Part print with two shaded views. Sizes in mm from the minimum x, y, z corner. A direction names the side the tool comes from. Round coordinates to 2 decimals unless told otherwise and drop trailing zeros. Write each loop counter-clockwise with the first axis right and the second up, starting at its lowest first coordinate (ties: lowest second). Pieces come first, ordered by that corner, then holes.
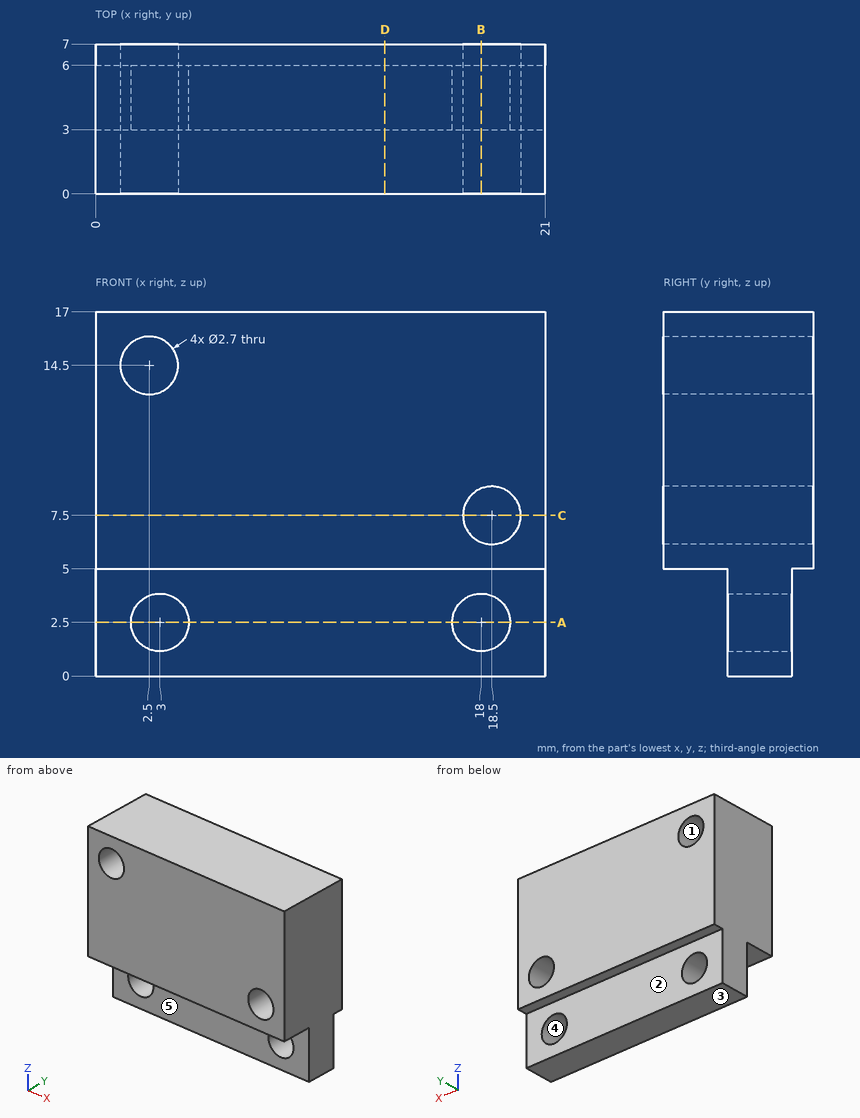
Q1. Cut at C-C on z = 7.5. Write the cut outline in (x, y), plus the area to 3 significant figures.
Values follow:
outline: (0, 0) - (17.15, 0) - (17.15, 7) - (0, 7) - close; (19.85, 0) - (21, 0) - (21, 7) - (19.85, 7) - close
area: 128 mm2
Q2. Cut at A-A on z = 2.5. Write the cut outline in (x, y).
Values follow:
outline: (0, 3) - (1.65, 3) - (1.65, 6) - (0, 6) - close; (4.35, 3) - (16.65, 3) - (16.65, 6) - (4.35, 6) - close; (19.35, 3) - (21, 3) - (21, 6) - (19.35, 6) - close
Q3. Mould opens along Z. For the marked faces 3, 4 and 5 say: +Z half, -Z half, draft (parallel to the pull), parting line (faces both ways), or undercut.
Values follow:
face 3: -Z half
face 4: undercut
face 5: draft
Q4. Cut at D-D on x = 13.5. Write the cut outline in (y, z).
Values follow:
outline: (0, 5) - (3, 5) - (3, 0) - (6, 0) - (6, 5) - (7, 5) - (7, 17) - (0, 17) - close
Q5. Which spindle directions (+Z, -Z, +X, -X, +Y, -Y) get a long thin tool onto all of the face, cutting with end or side? Do the marked faces 1 and 2. Say none if no direction does.
Values follow:
face 1: +Y, -Y
face 2: -Z, +X, -X, +Y
Q6. Cut at B-B on x = 18. Write the cut outline in (y, z), plus the area to 3 significant figures.
Values follow:
outline: (0, 5) - (3, 5) - (3, 3.85) - (6, 3.85) - (6, 5) - (7, 5) - (7, 6.25) - (0, 6.25) - close; (0, 8.75) - (7, 8.75) - (7, 17) - (0, 17) - close; (3, 0) - (6, 0) - (6, 1.15) - (3, 1.15) - close
area: 73.3 mm2
Q7. Drop flat-ended pins along their axis: pin 1 (3 mm diameter, centred on x = 18.5, z = 7.5, fed in from -Y); pin 2 (0.8 mm diameter, centred on x = 13, y = 6.5, fed in from -Z); pin 3 (1.5 mm diameter, centred on x = 12.5, z = 1.5, fed in from -Y); pin 4 (1.5 mm diameter, centred on x = 6, z = 2.5, fed in from +Y). Give the stop position or say it passes through.
Values follow:
pin 1: stops at y = 0
pin 2: stops at z = 5
pin 3: stops at y = 3
pin 4: stops at y = 6
Q8. Wall check: L1, parallel to X at y = 2.75, z = 14.5; L2, parallel to Z at x = 2.5, y = 2.5; L3, parallel to X at y = 5.75, z = 1.75. Give the ranges that are in metal, low to high.
Values follow:
L1: x = 0 to 1.15, 3.85 to 21
L2: z = 5 to 13.15, 15.85 to 17
L3: x = 0 to 1.88, 4.12 to 16.88, 19.12 to 21
